Geometry: final body of the model. Coordinates: model frame, mm. Face numbers are marked on the shaded views. A direction names the side the tool comes from. Round coordinates to 2 decimals unless told otherwise and drop trailing zeros. Loops run counter-clockwise (first coordinate to the right, second up) from the corner with the lowest first, then second, coordinate; pieces in that order, holes last. Notation, with made-up numbers: (7, 41) -> (45, 41) arc R28 cw to (45, 67) -> close; hole circle Ø6 at (48, 37). An arc over 180 degrees is marked (long way). Answer in a Markdown table with one row per item.
Autodesk Inventor part; units mm, degrees
ref_plane "YZ Plane" through (0, 0, 0) normal (1, 0, 0) x (0, 1, 0)
ref_plane "XZ Plane" through (0, 0, 0) normal (0, 1, 0) x (-1, 0, 0)
ref_plane "XY Plane" through (0, 0, 0) normal (0, 0, 1) x (1, 0, 0)
sketch "Sketch1" plane through (0, 0, 0) normal (0, 0, 1) x (1, 0, 0)
  line L0 (-14.0233, 19.5756) -> (11.3767, 19.5756)
  line L1 (11.3767, 19.5756) -> (11.3767, -5.8244)
  line L2 (11.3767, -5.8244) -> (-14.0233, -5.8244)
  line L3 (-14.0233, -5.8244) -> (-14.0233, 19.5756)
  line L4 (-10.8483, 16.4006) -> (8.2017, 16.4006)
  line L5 (8.2017, 16.4006) -> (8.2017, -2.6494)
  line L6 (8.2017, -2.6494) -> (-10.8483, -2.6494)
  line L7 (-10.8483, -2.6494) -> (-10.8483, 16.4006)
  point P0 (0, 0)
  dimension "d0" = 3.175
  dimension "d1" = 3.175
  dimension "d2" = 3.175
  dimension "d3" = 3.175
  dimension "d4" = 25.4
  dimension "d5" = 25.4
extrude "Extrusion1" add sketch "Sketch1" along normal blind 144.8308
equation "\"d1\" = d3"
equation "\"d2\" = d0"
equation "\"d3\" = d2"
equation "\"d5\" = d4"
properties part number "internalframeconnector"
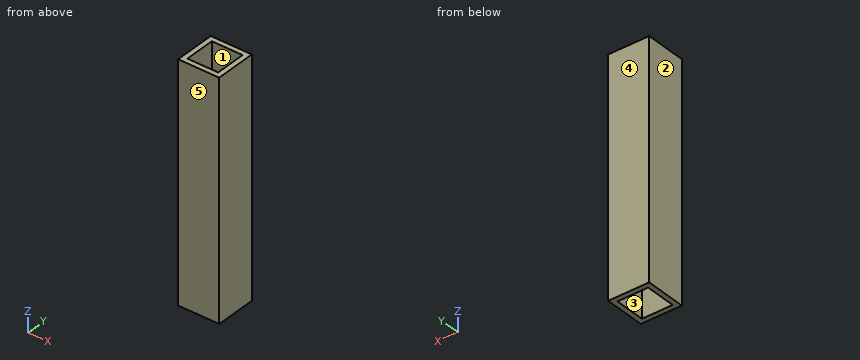
Item 1: Reachability of the marked faces 1 and 2 from +Z, -Z, +X, -X, +Y, -Y: full face, straight path, thin tool, end or side. Return the list, or none.
Answer:
| item | result |
|---|---|
| face 1 | +Z, -Z |
| face 2 | +Z, -Z, -X, +Y, -Y |
Item 2: Draft query along Y for the marked faces 3, 4 and 5. Return one class per face: pulls with the +Y half, pulls with the -Y half, needs draft (parallel to the pull), parting line crosses it, or undercut.
Answer:
| item | result |
|---|---|
| face 3 | undercut |
| face 4 | pulls with the +Y half |
| face 5 | pulls with the -Y half |
Item 3: Line query: probe 1 along X at (y, z) = (7.75, 53); probe 2 along Y at (x, z) = (-4.25, 35). Output: solid intervals per line, ascending. Write a range as [from, to].
Answer:
| item | result |
|---|---|
| probe 1 | x = [-14.02, -10.85], [8.2, 11.38] |
| probe 2 | y = [-5.82, -2.65], [16.4, 19.58] |
Item 4: Pin query (flat end, axial travel): pin 1 Ø12 at (x, y) = (-5.5, 9.5) entering from +Z; pin 2 Ø1 at (x, y) = (-2, -0.5) entering from -Z. Return the tip coordinate at first contact, or that it passes through.
Answer:
| item | result |
|---|---|
| pin 1 | stops at z = 144.83 |
| pin 2 | passes through |
Item 5: Cut plane A-A (y = 7.75). Output: boundary loops of the cut face in (x, z), then the cut area to 3 significant figures.
Answer:
| item | result |
|---|---|
| outline | (-14.02, 0) -> (-10.85, 0) -> (-10.85, 144.83) -> (-14.02, 144.83) -> close; (8.2, 0) -> (11.38, 0) -> (11.38, 144.83) -> (8.2, 144.83) -> close |
| area | 920 mm² |
Item 6: Cut plane B-B (z = 61). Output: boundary loops of the cut face in (x, y).
Answer:
| item | result |
|---|---|
| outline | (-14.02, -5.82) -> (11.38, -5.82) -> (11.38, 19.58) -> (-14.02, 19.58) -> close; hole (-10.85, -2.65) -> (8.2, -2.65) -> (8.2, 16.4) -> (-10.85, 16.4) -> close |
Item 7: Cut plane C-C (x = 7). Output: boundary loops of the cut face in (y, z).
Answer:
| item | result |
|---|---|
| outline | (-5.82, 0) -> (-2.65, 0) -> (-2.65, 144.83) -> (-5.82, 144.83) -> close; (16.4, 0) -> (19.58, 0) -> (19.58, 144.83) -> (16.4, 144.83) -> close |
